from build123d import *

# Parameters (mm, degrees)
SKETCH_1_W               = 4
SKETCH_1_H               = 7.5
CHAMFER_1_SIZE           = 0.5
HOLE_WIZARD_M4_1_D       = 3.3
PATTERN_CIRCULAR_1_COUNT = 8


with BuildPart() as part:
    # 草图1 → 旋转1 (revolve)
    with BuildSketch(Plane.XY, mode=Mode.PRIVATE) as revolve_1_sk:
        with Locations((2, 24.75)):
            Rectangle(SKETCH_1_W, SKETCH_1_H)
        Polygon((4, 21), (0, 21), (0, 18.5), (9.5, 18.5), (9.5, 21), align=None)
        Polygon((12.5, 21), (9.5, 21), (9.5, 18.5), (9.5, 16.25), (12.5, 16.25), align=None)
    revolve(revolve_1_sk.sketch.rotate(Axis((0, 0, 0), (1, 0, 0)), 90), axis=Axis((0, 0, 0), (1, 0, 0)))

    # 倒角1
    chamfer_1_edges = [part.edges().sort_by_distance(p)[0] for p in [
        (0, 0, -18.5),
        (0, 0, -28.5),
        (4, 0, -28.5),
        (12.5, 0, -16.25),
        (12.5, 0, -21),
    ]]
    chamfer(chamfer_1_edges, length=CHAMFER_1_SIZE)

    # M4 螺纹孔1 (through all)
    with Locations(Plane(origin=(4, 0, 0), x_dir=(0, 0, -1), z_dir=(1, 0, 0))):
        with Locations((0, 25)):
            hole_wizard_m4_1 = Hole(HOLE_WIZARD_M4_1_D / 2)

    # 阵列(圆周)1: M4 螺纹孔1 ×8 about axis
    pattern_circular_1_axis = Axis((0, 0, 0), (1, 0, 0))
    for i in range(1, PATTERN_CIRCULAR_1_COUNT):
        add(hole_wizard_m4_1.rotate(pattern_circular_1_axis, i * 360 / PATTERN_CIRCULAR_1_COUNT), mode=Mode.SUBTRACT)


solid = part.part
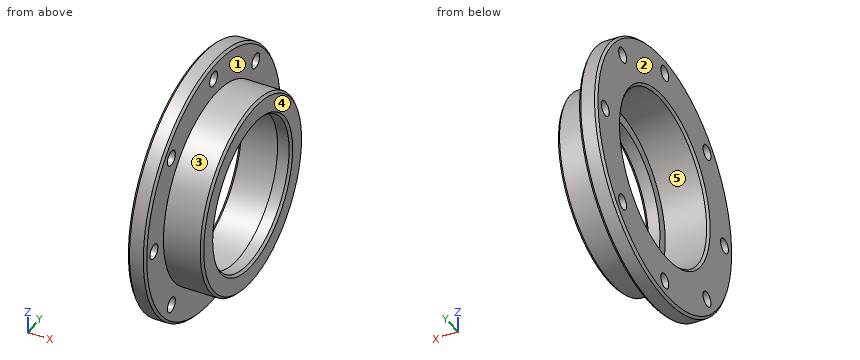
Check sheet for the modelled part. Datum: model origin and axes. Units: mm. Face numbers are marked on the shaded views. A direction names the side the tool comes from. Coordinates: 2 decimals unless noted, no trailing zeros. Write each loop counter-clockwise with the first axis right and the second up, starting at its lowest first coordinate (ties: lowest second). Pieces come first, ordered by that corner, then holes. Notation, with made-up numbers: M 67.5,76 L 112.5,76 A16 cw 112.5,104 Z; hole C 52,-12 d5. An arc over 180 degrees is marked long. Answer as CSV lines item,"result".
Q1. Go/stop test with flat-tipped pins: pin 1 (2.5 mm diameter, centred on y = 17.68, z = 17.68, fed in from -X); pin 2 (1.5 mm diameter, centred on x = 4.5, y = 6.5, fed in from -Z); pin 3 (4 mm diameter, centred on y = 0, z = -25, fed in from +X); pin 4 (4.5 mm diameter, centred on y = 17.68, z = -17.68, fed in from -X). Record where each tip stops, or that it passes through.
Check result:
pin 1,"through"
pin 2,"z = -27.51"
pin 3,"x = 4"
pin 4,"x = 0"
Q2. Cross-section at A-A (z = 0). Count the separate pieces of the cut face and the enclosed holes in it, then the cut area to 3 significant figures.
Check result:
separate pieces,"4"
enclosed holes,"0"
area,"108 mm^2"
Q3. Cross-section at C-C (x = 8.75). Record the boundary of the cut face in (y, z), then the cut area to 3 significant figures.
Check result:
outline,"C 0,0 d42; hole C 0,0 d37"
area,"310 mm^2"
Q4. Mould release check, pull along Y, two halves, no side actions. Record for the marked faces 3, 4 and 5: released by +Y, released by -Y, zero draft, split by the parting line, or undercut.
Check result:
face 3,"split by the parting line"
face 4,"zero draft"
face 5,"undercut"
Q5. Set-up check for the marked faces 1 and 2: record each of +Z, -Z, +X, -X, +Y, -Y from which the full face is reachable in a straight line by a thin tool's end or side.
Check result:
face 1,"+X"
face 2,"+Z, -Z, -X, +Y, -Y"
Q6. Material ranges on probe 1 along Y at (x, z) = (7.5, 0); probe 2 along X at (y, z) = (8, -20); probe 3 along Y at (x, z) = (10.5, -5), recorded low to high. Write a range as from..to.
Check result:
probe 1,"-21..-18.5, 18.5..21"
probe 2,"0..4"
probe 3,"-20.4..-15.46, 15.46..20.4"
